```python
from build123d import *

# Parameters (mm, degrees)
F1_DEPTH = 63.5
F0_W     = 25.4
F0_H     = 19.05
F2_DEPTH = 25.4
F3_DEPTH = 7.9375
F4_DEPTH = 25.4
F6_R     = 6.35


with BuildPart() as f1:
    # F0 (on Front) → F1 (new body, symmetric)
    with BuildSketch(Plane.XZ):
        Polygon((22.225, 9.525), (-41.275, 9.525), (-41.275, -9.525), (41.275, -9.525), (41.275, 9.525), align=None)
    extrude(amount=F1_DEPTH, both=True)

    # F0 (on Front) → F2 (join, symmetric)
    with BuildSketch(Plane.XZ):
        with Locations((73.025, 52.4002)):
            Rectangle(F0_W, F0_H)
        with BuildLine():
            Line((22.225, 27.0165912208), (22.225, 9.525))
            Line((22.225, 9.525), (41.275, 9.525))
            Line((41.275, 9.525), (41.275, 27.0165912208))
            ThreePointArc((41.275, 27.0165912208), (46.1826320332, 38.4940676368), (57.8712160479, 42.8752))
            Line((57.8712160479, 42.8752), (60.325, 42.8752))
            Line((60.325, 42.8752), (60.325, 61.9252))
            Line((60.325, 61.9252), (58.2198869565, 61.9252))
            add(Edge.make_bspline(
                [(54.2612726793, 61.8219195408), (55.5968119666, 61.8785577598), (56.917161192, 61.9131437071), (58.2198869565, 61.9252)],
                knots=[108.8449381095, 108.8449381095, 108.8449381095, 108.8449381095, 112.4500488685, 112.4500488685, 112.4500488685, 112.4500488685], degree=3))
            ThreePointArc((54.2612726793, 61.8219195408), (31.4532645393, 50.66893596), (22.225, 27.0165912208))
        make_face()
    extrude(amount=F2_DEPTH, both=True)

    # F0 (on Front) → F3 (join, symmetric)
    with BuildSketch(Plane.XZ):
        with BuildLine():
            add(Edge.make_bspline(
                [(-41.275, 9.525), (-40.2299736502, 38.3002045249), (13.9388801659, 60.1119073253), (54.2612726793, 61.8219195408)],
                knots=[0, 0, 0, 0, 108.8449381095, 108.8449381095, 108.8449381095, 108.8449381095], degree=3))
            Line((-41.275, 9.525), (22.225, 9.525))
            Line((22.225, 9.525), (22.225, 27.0165912208))
            ThreePointArc((22.225, 27.0165912208), (31.4532645393, 50.66893596), (54.2612726793, 61.8219195408))
        make_face()
    extrude(amount=F3_DEPTH, both=True)

    # F0 (on Front) → F4 (join, symmetric)
    with BuildSketch(Plane.XZ):
        with Locations((73.025, 52.4002)):
            Rectangle(F0_W, F0_H)
    extrude(amount=F4_DEPTH, both=True)

    # F0 (on Front) → F5 (revolve)
    with BuildSketch(Plane.XZ):
        Polygon((85.725, 66.675), (85.725, 61.9252), (85.725, 42.8752), (85.725, 38.1), (111.125, 38.1), (111.125, 66.675), align=None)
    revolve(axis=Axis((85.725, 0, 52.3875), (0, 0, -1)))

    # F6
    f6_edges = [f1.edges().sort_by_distance(p)[0] for p in [
        (-41.275, -63.5, 0),
        (41.275, -63.5, 0),
        (41.275, 63.5, 0),
        (-41.275, 63.5, 0),
    ]]
    fillet(f6_edges, radius=F6_R)


solid = f1.part
```
The listing builds one solid part. Answer for the finished solid, in the listing's coordinates (mm). A direction names the side the tool comes from. Round coordinates to 2 decimals unless told otherwise and drop trailing zeros. Write each loop counter-clockwise with the first axis right and the second up, starting at its lowest first coordinate (ties: lowest second). Pieces come first, ordered by that corner, then holes. Notation, with made-up numbers: (18, 70) -> (73, 70) arc R31 cw to (73, 102) -> close; hole circle Ø3 at (-33.5, -14.5). An arc over 180 degrees is marked (long way). Answer as a JSON object with one key per item and string values. Group by question number.
Q1. Section A-A (z = -3) is taken. Write down the section's boundary in (x, y) (3 decimals), plus the area to 3 significant figures.
Q2. Which of the six approach directions +Z, -Z, +X, -X, +Y, -Y give full straight-line access (tool end or side, diameter ignored) to faces 1 (the face through (31.701, 16.547, 50.935)), 2 (the face through (41.275, -1, 4)), 3 (the face through (46, 25.4, 42)), 4 (the face through (-3, -7.938, 30))?
Q3. Each of these flat-tipped pins is pushed along its axis until it touches: pin 1 Ø14 at (x, y) = (76, 4) entering from -Z; pin 2 Ø16.5 at (x, y) = (-4, 25.5) entering from +Z (3 decimals); pin 3 Ø5 at (y, z) = (40, -1.5) entering from +X (3 decimals); pin 4 Ø1.5 at (x, z) = (43.5, 6.5) entering from -Y. Where does it stop, or does it pass through?
Q4. Straight lines are drawn through the part: line 1 along Z through (x, y) = (8, -37) (3 decimals); line 2 along Y through (x, z) = (-14.5, 12); line 3 along Y through (x, z) = (55, 44). For each, find the intervals that lie inside material, in ascending order.
Q5. Section B-B (y = 44) is taken. Write down the section's boundary in (x, z) (3 decimals), plus the area to 3 significant figures.
Check values:
{
 "1": {"outline": "(-41.275, -57.15) arc R6.35 ccw to (-34.925, -63.5) -> (34.925, -63.5) arc R6.35 ccw to (41.275, -57.15) -> (41.275, 57.15) arc R6.35 ccw to (34.925, 63.5) -> (-34.925, 63.5) arc R6.35 ccw to (-41.275, 57.15) -> close", "area": "10,400 mm^2"},
 "2": {"face 1": "+Z, -X, +Y", "face 2": "-Z, +X, +Y, -Y", "face 3": "+Z, +X, -X, +Y", "face 4": "+Z, -X, -Y"},
 "3": {"pin 1": "z = 38.1", "pin 2": "z = 9.525", "pin 3": "x = 41.275", "pin 4": "through"},
 "4": {"line 1": "-9.525 to 9.525", "line 2": "-7.94 to 7.94", "line 3": "-25.4 to 25.4"},
 "5": {"outline": "(-41.275, -9.525) -> (41.275, -9.525) -> (41.275, 9.525) -> (-41.275, 9.525) -> close", "area": "1,570 mm^2"}
}
